```python
from build123d import *

# Parameters (mm, degrees)
SKETCH1_R           = 37.5
SKETCH1_R_2         = 33.5
BOSS_EXTRUDE1_DEPTH = 800


with BuildPart() as part:
    # Sketch1 → Boss-Extrude1 (new body)
    with BuildSketch(Plane(origin=(0, 0, 0), x_dir=(1, 0, 0), z_dir=(0, 1, 0))):
        with Locations(Location((0, 0, 0), (0, 0, 270))):
            Circle(SKETCH1_R)
        with Locations(Location((0, 0, 0), (0, 0, 270))):
            Circle(SKETCH1_R_2, mode=Mode.SUBTRACT)
    extrude(amount=BOSS_EXTRUDE1_DEPTH)

    # Sketch2 → Revolve1 (revolve)
    with BuildSketch(Plane(origin=(0, 0, 0), x_dir=(0, 0, -1), z_dir=(1, 0, 0)), mode=Mode.PRIVATE) as revolve1_sk:
        Polygon((-33.5, 650), (-30.5, 660), (-33.5, 660), align=None)
    revolve(revolve1_sk.sketch.rotate(Axis((0, 800, 0), (0, -1, 0)), 180), axis=Axis((0, 800, 0), (0, -1, 0)))


solid = part.part
```
CAD build for the part. Positions are in the model's coordinates, mm. A direction names the side the tool comes from. Round coordinates to 2 decimals unless told otherwise and drop trailing zeros. Loops run counter-clockwise (first coordinate to the right, second up) from the corner with the lowest first, then second, coordinate; pieces in that order, holes last. Notation, with made-up numbers: M 75.5,80 L 105.5,80 A30 cw 105.5,103 Z; hole C -19,-38.5 d5. An arc over 180 degrees is marked long. Return JSON: item names as keys, results as strings. Group by question number.
(1) Saw through at A-A, the plane z = 0. List the corners of the cut face in (x, y).
(2) Mould opens along X. For faces 1 (the flat face through (-30, 660, 7)), 2 (the flat face through (31, 0, -14)), 3 (the cylindrical face through (-22.818, 394.4, -29.759)) say: +X half, -X half, draft (parallel to the pull), parting line (faces both ways), or undercut.
(3) Tool access for faces 4 (the cylindrical face through (-29.7, 729, 15.5)), 5 (the flat face through (31, 800, -14)), 6 (the cylindrical face through (-29.7, 320.4, 15.5)): list every direction of +Z, -Z, +X, -X, +Y, -Y with a clear straight run to the whole face (end or side of a thin tool).
(4) Saw through at B-B, the plane x = 0. List the corners of the cut face in (y, z).
(5) Drop flat-ended pins along their axis: P1, Ø4, axis at y = 432.5, z = -8, coming from the -X side; P2, Ø1, axis at x = 12.5, y = 457, coming from the -Z side; P3, Ø1.5, axis at y = 621, z = -25.5, coming from the -X side; P4, Ø4, axis at x = 27.5, z = 18, coming from the +Y side. Give the stop position or say it passes through.
(6) Saw through at C-C, the plane y = 196. List the corners of the cut face in (x, z).
(7) Wall check: probe 1 along X at (y, z) = (284, 0); probe 2 along Z at (x, y) = (2, 398). Give the ranges that are in metal, low to high. Write a range as [from, to].
Answer list:
{
 "1": {"outline": "M -37.5,0 L -33.5,0 L -33.5,650 L -30.5,660 L -33.5,660 L -33.5,800 L -37.5,800 Z; M 30.5,660 L 33.5,650 L 33.5,0 L 37.5,0 L 37.5,800 L 33.5,800 L 33.5,660 Z"},
 "2": {"face 1": "undercut", "face 2": "draft", "face 3": "parting line"},
 "3": {"face 4": "+Y", "face 5": "+Z, -Z, +X, -X, +Y", "face 6": "-Y"},
 "4": {"outline": "M 0,-37.5 L 800,-37.5 L 800,-33.5 L 660,-33.5 L 660,-30.5 L 650,-33.5 L 0,-33.5 Z; M 0,33.5 L 650,33.5 L 660,30.5 L 660,33.5 L 800,33.5 L 800,37.5 L 0,37.5 Z"},
 "5": {"P1": "x = -37.02", "P2": "z = -35.53", "P3": "x = -28.17", "P4": "y = 800"},
 "6": {"outline": "C 0,0 d75; hole C 0,0 d67"},
 "7": {"probe 1": "[-37.5, -33.5], [33.5, 37.5]", "probe 2": "[-37.45, -33.44], [33.44, 37.45]"}
}
